from build123d import *

# Parameters (mm, degrees)
SKETCH_1_W          = 70
SKETCH_1_H          = 40
EXTRUDE_1_DEPTH     = 30
SKETCH_6_W          = 25
SKETCH_6_H          = 16
CUT_EXTRUDE_2_DEPTH = 87.02325267
EXTRUDE_6_DEPTH     = 25
SKETCH_10_R         = 5
CUT_EXTRUDE_4_DEPTH = 95.868329805


with BuildPart() as part:
    # 草图1 → 凸台-拉伸1 (new body)
    with BuildSketch(Plane(origin=(0, 0, 0), x_dir=(1, 0, 0), z_dir=(0, 1, 0))):
        with Locations((35, -20)):
            Rectangle(SKETCH_1_W, SKETCH_1_H)
    extrude(amount=EXTRUDE_1_DEPTH)

    # 草图6 → 切除-拉伸2 (cut, through all)
    with BuildSketch(Plane(origin=(0, 30, 0), x_dir=(1, 0, 0), z_dir=(0, 1, 0))):
        with Locations((57.5, -20)):
            Rectangle(SKETCH_6_W, SKETCH_6_H)
    extrude(amount=-CUT_EXTRUDE_2_DEPTH, mode=Mode.SUBTRACT)

    # 草图9 → 凸台-拉伸6 (add)
    with BuildSketch(Plane(origin=(0, 0, 0), x_dir=(0, 0, -1), z_dir=(1, 0, 0))):
        Polygon((0, 0), (-40, 0), (-40, 30), (-20, 50), (0, 50), align=None)
    extrude(amount=EXTRUDE_6_DEPTH)

    # 草图10 → 切除-拉伸4 (cut, through all)
    with BuildSketch(Plane(origin=(0, 0, 0), x_dir=(0, 0, -1), z_dir=(1, 0, 0))):
        with Locations(Location((-12, 35, 0), (0, 0, 270))):
            Circle(SKETCH_10_R)
    extrude(amount=CUT_EXTRUDE_4_DEPTH, mode=Mode.SUBTRACT)


solid = part.part
Could you check a few things on this model? Use its own coordinates, in mm. A direction names the side the tool comes from. Coordinates: 2 decimals unless noted, no trailing zeros. Loops run counter-clockwise (first coordinate to the right, second up) from the corner with the lowest first, then second, coordinate; pieces in that order, holes last.
1. For P1, Ø10, axis at y = 8, z = 22.5, coming from the +X side; P2, Ø6, axis at y = 36.5, z = 16, coming from the +X side; P3, Ø20, axis at x = 42.5, z = 12, coming from the +Y side, each with a flat end and sliding along its axis, tell me the tip position at first contact or that it passes through.
2. For faces 1 (the face through (12, 50, 10)), 2 (the face through (25, 40, 15)), 3 (the face through (45, 15, 20)), which set-ups out of +Z, -Z, +X, -X, +Y, -Y let a thin tool reach every point of the face, with its end or its side?
3. Imagine slicing it at D-D (y = 18). Please give me the cut outline in (x, z), and give its area (3 significant figures).
4. Imagine slicing it at B-B (z = 10). Please give me the cut outline in (x, y), and give its area (3 significant figures).
5. I need wall thicknesses on L1, parallel to Z at x = 53, y = 20.5; L2, parallel to Z at x = 15.25, y = 35; L3, parallel to X at y = 10, z = 26.5. Which ranges of each line are inside material? Lowest first, please.
6. We'd pull the mould along Z, two halves only. Please class faces 4 (the face through (12, 40, 12)), 5 (the face through (70, 15, 34)), 6 (the face through (27, 19, 0)): released by +Z, released by -Z, zero draft, split by the parting line, or undercut.
7. Imagine slicing it at A-A (y = 31). Please give me the cut outline in (x, z).
8. Imagine slicing it at C-C (x = 8). Please give me the cut outline in (y, z).
Computed values:
1. P1: stops at x = 45
1. P2: stops at x = 25
1. P3: stops at y = 30
2. face 1: +Z, -Z, +X, -X, +Y
2. face 2: +Z, -Z, +X, +Y
2. face 3: +X, +Y, -Y
3. outline: (0, 0) - (70, 0) - (70, 12) - (45, 12) - (45, 28) - (70, 28) - (70, 40) - (0, 40) - close
3. area: 2,400 mm2
4. outline: (0, 0) - (70, 0) - (70, 30) - (25, 30) - (25, 30.42) - (0, 30.42) - close; (0, 39.58) - (25, 39.58) - (25, 50) - (0, 50) - close
4. area: 2,370 mm2
5. L1: z = 0 to 12, 28 to 40
5. L2: z = 0 to 7, 17 to 35
5. L3: x = 0 to 45
6. face 4: undercut
6. face 5: zero draft
6. face 6: released by -Z
7. outline: (0, 0) - (25, 0) - (25, 9) - (0, 9) - close; (0, 15) - (25, 15) - (25, 39) - (0, 39) - close
8. outline: (0, 0) - (50, 0) - (50, 20) - (30, 40) - (0, 40) - close; hole circle Ø10 at (35, 12)
